Input: part model. Units: mm. Frame: model coordinates. A direction names the side the tool comes from. Give positions to 0.01 mm unless a question says otherwise; leave off trailing zeros. Loops run counter-clockwise (first coordinate to the right, second up) from the corner with the lowest first, then second, coordinate; pieces in that order, holes last. Notation, with made-up numbers: (48, -10.5) - (68, -10.5) arc R23 ccw to (68, -1.5) - close; hole circle Ø8 at (37.5, 7). An arc over 180 degrees is marked (long way). Answer as a JSON object with one key per item and string values. Group by question number.
(1) Section query A-A (x = 137.5). Return loops of the section in (y, z), plus the area to 3 significant figures.
(2) Access query for faces 5 (the cylindrical face through (199.493, 2.03, 2.214)), 6 (the cylindrical face through (-199.49, -2.93, -0.65)), 7 (the flat face through (-198, 2, -2)), 8 (the cylindrical face through (2.744, -1.341, -3.233)). Directions: +Z, -Z, +X, -X, +Y, -Y. A direction counts if a zero-diameter tool reaches every point of the face in a straight line with its end or side. Return the directions, or none.
(3) Material intervals for L1, parallel to X at y = -0.75, z = 3.25; L2, parallel to X at y = -0.75, z = 2.75; L3, parallel to Y at x = -142, z = 0.25, sorted ascending.
(4) Pin query (flat end, axial travel): P1, Ø3, axis at x = -158.5, y = 2, coming from the -Z side; P2, Ø4, axis at x = 87.5, z = 2.5, coming from the +Y side; P3, Ø1.5, axis at x = -78.5, z = 1.5, coming from the +Y side. Return the tip coordinate at first contact, or that it passes through.
(5) Mould query, pull axis X, two halves, no side actions, for faces 1 (the flat face through (196, 1, -3)), 2 (the flat face through (-200, 0, 0)), 3 (the flat face through (197, 1, -3)), 4 (the cylindrical face through (-197.493, 1.341, -3.233)). Classes: +X half, -X half, draft (parallel to the pull), parting line (faces both ways), or undercut.
```python
from build123d import *

# Parameters (mm, degrees)
SKETCH1_R            = 3.5
BOSS_EXTRUDE1_DEPTH  = 196
SKETCH6_R            = 2.999428485
BOSS_EXTRUDE4_DEPTH  = 1
BOSS_EXTRUDE5_START  = 1
SKETCH7_R            = 3.5
BOSS_EXTRUDE5_DEPTH  = 1
SKETCH8_R            = 2.50271342
BOSS_EXTRUDE6_DEPTH  = 1
SKETCH9_R            = 3.004216162
BOSS_EXTRUDE7_DEPTH  = 1
SKETCH10_R           = 2.999964983
BOSS_EXTRUDE8_DEPTH  = 1
SKETCH11_R           = 3.5
BOSS_EXTRUDE9_DEPTH  = 1
SKETCH12_R           = 2.504776308
BOSS_EXTRUDE10_DEPTH = 1
SKETCH13_R           = 3.002711456
BOSS_EXTRUDE11_DEPTH = 1


with BuildPart() as part:
    # Sketch1 → Boss-Extrude1 (new, symmetric)
    with BuildSketch(Plane(origin=(0, 0, 0), x_dir=(0, 0, -1), z_dir=(1, 0, 0))):
        Circle(SKETCH1_R)
    extrude(amount=BOSS_EXTRUDE1_DEPTH, both=True)

    # Sketch6 → Boss-Extrude4 (add)
    with BuildSketch(Plane(origin=(196, 0, 0), x_dir=(0, 0, -1), z_dir=(1, 0, 0))):
        Circle(SKETCH6_R)
    extrude(amount=BOSS_EXTRUDE4_DEPTH)

    # Sketch7 → Boss-Extrude5 (add)
    with BuildSketch(Plane(origin=(197, 0, 0), x_dir=(0, 0, -1), z_dir=(1, 0, 0)).offset(BOSS_EXTRUDE5_START)):
        Circle(SKETCH7_R)
    extrude(amount=-BOSS_EXTRUDE5_DEPTH)

    # Sketch8 → Boss-Extrude6 (add)
    with BuildSketch(Plane(origin=(198, 0, 0), x_dir=(0, 0, -1), z_dir=(1, 0, 0))):
        Circle(SKETCH8_R)
    extrude(amount=BOSS_EXTRUDE6_DEPTH)

    # Sketch9 → Boss-Extrude7 (add)
    with BuildSketch(Plane(origin=(199, 0, 0), x_dir=(0, 0, -1), z_dir=(1, 0, 0))):
        Circle(SKETCH9_R)
    extrude(amount=BOSS_EXTRUDE7_DEPTH)

    # Sketch10 → Boss-Extrude8 (add)
    with BuildSketch(Plane.ZY.offset(196)):
        Circle(SKETCH10_R)
    extrude(amount=BOSS_EXTRUDE8_DEPTH)

    # Sketch11 → Boss-Extrude9 (add)
    with BuildSketch(Plane.ZY.offset(197)):
        with Locations(Location((0, 0, 0), (0, 0, 180))):
            Circle(SKETCH11_R)
    extrude(amount=BOSS_EXTRUDE9_DEPTH)

    # Sketch12 → Boss-Extrude10 (add)
    with BuildSketch(Plane.ZY.offset(198)):
        Circle(SKETCH12_R)
    extrude(amount=BOSS_EXTRUDE10_DEPTH)

    # Sketch13 → Boss-Extrude11 (add)
    with BuildSketch(Plane.ZY.offset(199)):
        Circle(SKETCH13_R)
    extrude(amount=BOSS_EXTRUDE11_DEPTH)


solid = part.part
```
Recorded:
{
 "1": {"outline": "circle Ø7 at (0, 0)", "area": "38.5 mm^2"},
 "2": {"face 5": "+X", "face 6": "-X", "face 7": "none", "face 8": "+X, -X"},
 "3": {"L1": "x = -198 to -197, -196 to 196, 197 to 198", "L2": "x = -200 to -199, -198 to 198, 199 to 200", "L3": "y = -3.49 to 3.49"},
 "4": {"P1": "stops at z = -3.46", "P2": "stops at y = 3.46", "P3": "stops at y = 3.42"},
 "5": {"face 1": "undercut", "face 2": "-X half", "face 3": "undercut", "face 4": "draft"}
}
